```python
from build123d import *

# Parameters (mm, degrees)
SKETCH1_R           = 2.286
BOSS_EXTRUDE1_DEPTH = 1.5875


with BuildPart() as part:
    # Sketch1 → Boss-Extrude1 (new body)
    with BuildSketch(Plane(origin=(0, 0, 0), x_dir=(1, 0, 0), z_dir=(0, 1, 0))):
        Polygon((-154.686, -36.195), (-154.686, 6.985), (-182.708271591, 6.985), (-182.708271591, 36.195), (182.708271591, 36.195), (182.708271591, 6.985), (154.686, 6.985), (154.686, -36.195), align=None)
        with Locations(Location((175.1457, 17.78, 0), (0, 0, 270))):
            Circle(SKETCH1_R, mode=Mode.SUBTRACT)
        with Locations(Location((0, 29.845, 0), (0, 0, 270))):
            Circle(SKETCH1_R, mode=Mode.SUBTRACT)
        with Locations(Location((146.177, -33.02, 0), (0, 0, 270))):
            Circle(SKETCH1_R, mode=Mode.SUBTRACT)
        with Locations(Location((-175.1457, 17.78, 0), (0, 0, 270))):
            Circle(SKETCH1_R, mode=Mode.SUBTRACT)
        with Locations(Location((0, -33.02, 0), (0, 0, 270))):
            Circle(SKETCH1_R, mode=Mode.SUBTRACT)
        with Locations(Location((-146.177, -33.02, 0), (0, 0, 270))):
            Circle(SKETCH1_R, mode=Mode.SUBTRACT)
    extrude(amount=BOSS_EXTRUDE1_DEPTH)


solid = part.part
```
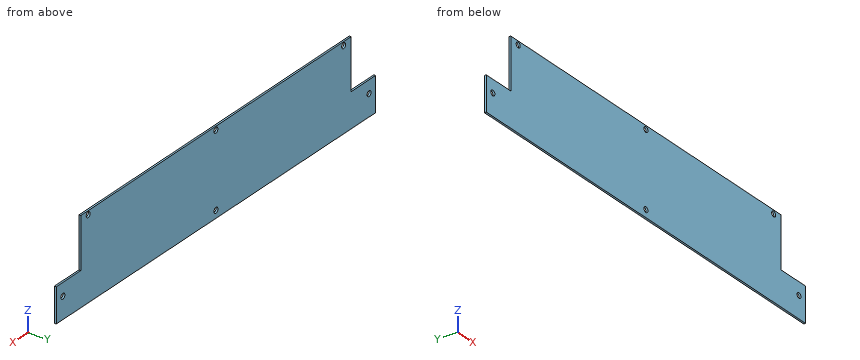
Verification items for the finished model (mm, model axes). Coordinates: 2 decimals unless noted, no trailing zeros. Write each loop counter-clockwise with the first axis right and the second up, starting at its lowest first coordinate (ties: lowest second). Pieces come first, ordered by that corner, then holes. Notation, with made-up numbers: M 60.25,22.5 L 80.25,22.5 A26 cw 80.25,50.5 Z; hole C -14.5,51 d8. An arc over 180 degrees is marked long. Answer as a JSON object with one key per item and string values. Group by question number.
(1) Material ranges on line 1 (X direction, y = 0.75, z = 33.02); line 2 (X direction, y = 0.35, z = -17.5); line 3 (X direction, y = 1, z = -29.5), recorded low to high.
(2) Gauge pin test, flat end, axial feed: pin 1 (0.5 mm diameter, centred on x = -167, y = 0.5, fed in from +Z) (3 decimals). Record the tip position at first contact, or that the pin passes through.
(3) Cross-section at B-B, the plane z = 3.5. Record the cut outline in (x, y).
(4) Cross-section at A-A, the plane y = 0.6. Record the cut outline in (x, z) (3 decimals).
Reply:
{
 "1": {"line 1": "-154.69 to -148.46, -143.89 to -2.29, 2.29 to 143.89, 148.46 to 154.69", "line 2": "-182.71 to -177.41, -172.88 to 172.88, 177.41 to 182.71", "line 3": "-182.71 to -2.26, 2.26 to 182.71"},
 "2": {"pin 1": "z = -6.985"},
 "3": {"outline": "M -154.69,0 L 154.69,0 L 154.69,1.59 L -154.69,1.59 Z"},
 "4": {"outline": "M -182.708,-36.195 L 182.708,-36.195 L 182.708,-6.985 L 154.686,-6.985 L 154.686,36.195 L -154.686,36.195 L -154.686,-6.985 L -182.708,-6.985 Z; hole C -175.146,-17.78 d4.572; hole C -146.177,33.02 d4.572; hole C 0,-29.845 d4.572; hole C 0,33.02 d4.572; hole C 146.177,33.02 d4.572; hole C 175.146,-17.78 d4.572"}
}
